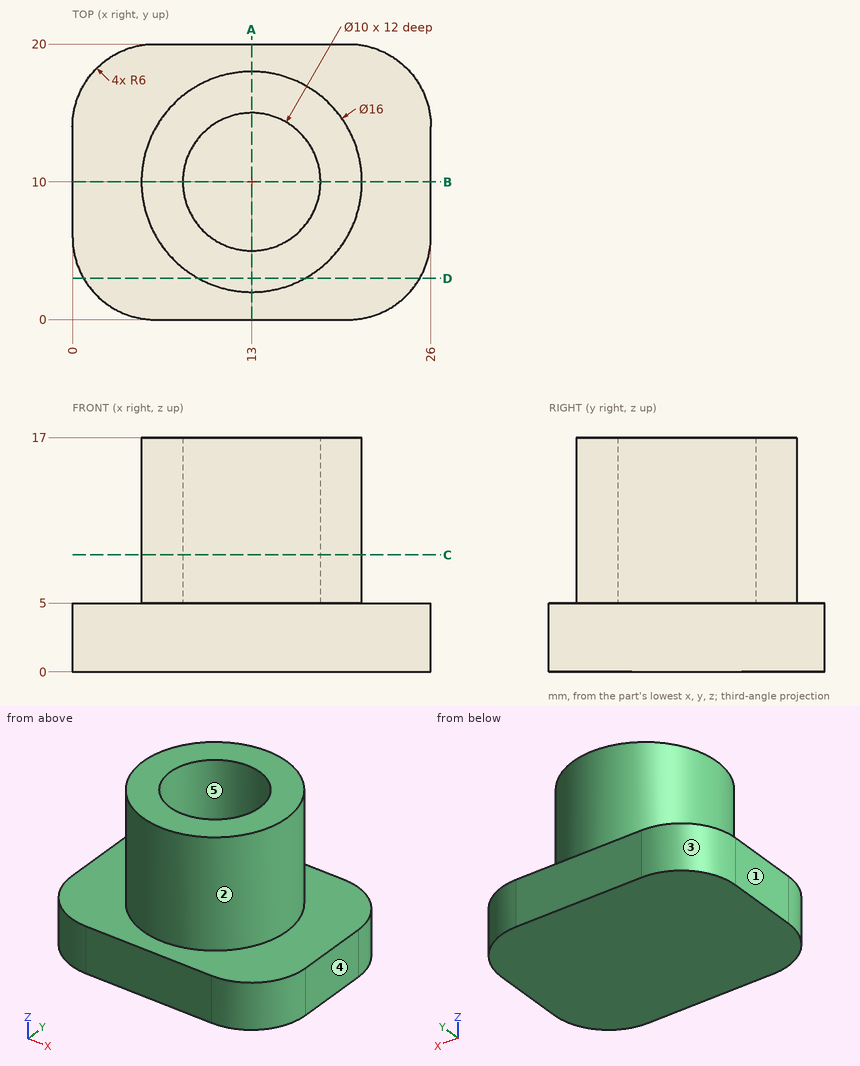
Job drawing, mm, ordinate dimensions from the low corner. One solid piece. A direction names the side the tool comes from. Give positions to 0.01 mm unless a question says otherwise; leave off trailing zeros. Loops run counter-clockwise (first coordinate to the right, second up) from the corner with the lowest first, then second, coordinate; pieces in that order, holes last.
Item 1: Slice it at B-B, the plane y = 10. List the corners of the cut face in (x, z).
Answers follow:
outline: (0, 0) - (26, 0) - (26, 5) - (21, 5) - (21, 17) - (18, 17) - (18, 5) - (8, 5) - (8, 17) - (5, 17) - (5, 5) - (0, 5) - close
Item 2: Drill centre lines: line 1 (Y direction, x = 13, z = 14); line 2 (Z direction, x = 11, y = 7.5); line 3 (Y direction, x = 14.5, z = 5.5). Where is each one in solid material? Low to high.
Answers follow:
line 1: y = 2 to 5, 15 to 18
line 2: z = 0 to 5
line 3: y = 2.14 to 5.23, 14.77 to 17.86
Item 3: Slice it at A-A, the plane x = 13. List the corners of the cut face in (y, z).
Answers follow:
outline: (0, 0) - (20, 0) - (20, 5) - (18, 5) - (18, 17) - (15, 17) - (15, 5) - (5, 5) - (5, 17) - (2, 17) - (2, 5) - (0, 5) - close
Item 4: Pull direction X, two halves, no side cores. Call the marked faces 3, 4 and 5: released by +X, released by -X, zero draft, split by the parting line, or undercut.
Answers follow:
face 3: released by -X
face 4: released by +X
face 5: undercut
Item 5: Slice it at C-C, the plane z = 8.5. List the corners of the cut face in (x, y), and give its area (3 significant figures).
Answers follow:
outline: circle Ø16 at (13, 10); hole circle Ø10 at (13, 10)
area: 123 mm2
Item 6: Which spindle directions (+Z, -Z, +X, -X, +Y, -Y) get a long thin tool onto all of the face, cutting with end or side? Do the marked faces 1 and 2. Say none if no direction does.
Answers follow:
face 1: +Z, -Z, -X, +Y, -Y
face 2: +Z
Item 7: Flat gauge pins, fed straight in: pin 1 (4 mm diameter, centred on x = 12, z = 8.5, fed in from -Y); pin 2 (8 mm diameter, centred on y = 3, z = 12, fed in from -X); pin 3 (8 mm diameter, centred on x = 13, y = 10, fed in from +Z). Where does each tip first touch, or does it go through?
Answers follow:
pin 1: stops at y = 2
pin 2: stops at x = 5.58
pin 3: stops at z = 5
Item 8: Slice it at D-D, the plane y = 3. List the corners of the cut face in (x, z), and give its area (3 significant figures).
Answers follow:
outline: (0.8, 0) - (25.2, 0) - (25.2, 5) - (16.87, 5) - (16.87, 17) - (9.13, 17) - (9.13, 5) - (0.8, 5) - close
area: 215 mm2
